Answer from the drawing. Dimensions are ordinates in mm from the lowest x, y and z of the part. Coordinates: 2 decimals unless noted, no trailing zeros. Write each loop counter-clockwise with the first axis right and the second up, starting at its lowest first coordinate (ties: lowest second). Pieces come first, ordered by that corner, then holes. Notation, with made-up numbers: (16, 45) -> (51, 45) arc R14 ccw to (51, 69) -> close; hole circle Ø4 at (26.5, 18). An arc over 180 degrees is marked (long way). Return JSON: item names as keys, results as strings.
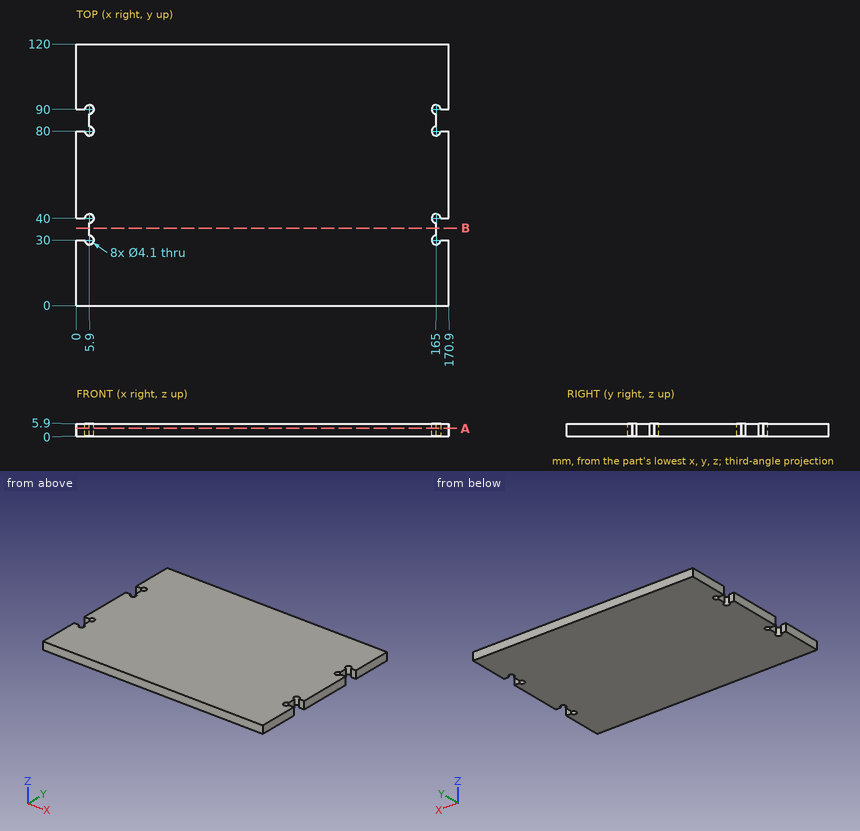
1. The part is cut by section B-B (y = 35.5). Determine the outline of the cut face in (x, z).
Taken from the geometry:
{"outline": "(5.9, 0) -> (165, 0) -> (165, 5.9) -> (5.9, 5.9) -> close"}
2. Consider L1, parallel to X at y = 36, z = 1.6. Determine where the line is inside the solid, lowest interval first.
Taken from the geometry:
{"L1": "x = 5.9 to 165"}
3. Flat-ended cylindrical pins translate along their axes: pin 1 Ø2.5 at (x, y) = (165, 40) entering from +Z; pin 2 Ø1.8 at (y, z) = (84, 3.5) entering from -X. Find the tip coordinate at first contact, or state that the pin passes through.
Taken from the geometry:
{"pin 1": "passes through", "pin 2": "stops at x = 5.9"}
4. The part is cut by section A-A (z = 3.65). Determine the outline of the cut face in (x, y).
Taken from the geometry:
{"outline": "(0, 0) -> (170.9, 0) -> (170.9, 30) -> (167.05, 30) arc R2.05 cw (long way) to (165, 32.05) -> (165, 37.95) arc R2.05 cw (long way) to (167.05, 40) -> (170.9, 40) -> (170.9, 80) -> (167.05, 80) arc R2.05 cw (long way) to (165, 82.05) -> (165, 87.95) arc R2.05 cw (long way) to (167.05, 90) -> (170.9, 90) -> (170.9, 120) -> (0, 120) -> (0, 90) -> (3.85, 90) arc R2.05 cw (long way) to (5.9, 87.95) -> (5.9, 82.05) arc R2.05 cw (long way) to (3.85, 80) -> (0, 80) -> (0, 40) -> (3.85, 40) arc R2.05 cw (long way) to (5.9, 37.95) -> (5.9, 32.05) arc R2.05 cw (long way) to (3.85, 30) -> (0, 30) -> close"}
